Autodesk Inventor part; units mm, degrees
ref_plane "YZ Plane" through (0, 0, 0) normal (1, 0, 0) x (0, 1, 0)
ref_plane "XZ Plane" through (0, 0, 0) normal (0, 1, 0) x (-1, 0, 0)
ref_plane "XY Plane" through (0, 0, 0) normal (0, 0, 1) x (1, 0, 0)
sketch "Sketch1" plane through (0, 0, 0) normal (0, 1, 0) x (-1, 0, 0)
  line L0 (12.7, -31.75) -> (-12.7, -31.75)
  line L1 (-12.7, -31.75) -> (-12.7, 31.75)
  line L2 (-12.7, 31.75) -> (12.7, 31.75)
  line L3 (12.7, 31.75) -> (12.7, -31.75)
  line L4 (12.7, -31.75) -> (-12.7, 31.75) construction
  line L5 (-12.7, -31.75) -> (12.7, 31.75) construction
  line L6 (-5.5118, -31.75) -> (-5.5118, 31.75)
  line L7 (12.7, 0) -> (-12.7, 0)
  circle A0 centre (-5.5118, 24.5618) radius 3.5052
  circle A1 centre (-5.5118, -24.5618) radius 3.5052
  line L8 (88.6284, 0) -> (-89.1716, 0)
  circle A2 centre (-30.9118, 0) radius 3.81
  line L9 (12.7, 31.75) -> (-12.7, 31.75)
  circle A3 centre (-30.9118, 0) radius 10.9982
  point P0 (0, 0)
  dimension "d0" = 25.4
  dimension "d1" = 63.5
  dimension "d2" = 7.1882
  dimension "d3" = 7.1882
  dimension "d4" = 7.0104
  dimension "d5" = 7.62
  dimension "d6" = 177.8
  dimension "d7" = 0
  dimension "d8" = 25.4
  dimension "d10" = 7.1882
extrude "Extrusion1" add sketch "Sketch1" along normal blind 5
sketch "Sketch2" plane through (0, 5, 0) normal (0, 1, 0) x (1, 0, 0)
  line L0 (12.7, -31.75) -> (38.3668, -8.086)
  circle A0 centre (30.9118, 0) radius 10.9982
  circle A1 centre (30.9118, 0) radius 10.9982
  line L1 (-12.7, 31.75) -> (-12.7, -31.75)
  line L2 (-12.7, 0) -> (12.7, 0)
  line L3 (12.7, -31.75) -> (12.7, 31.75)
  line L4 (12.7, 31.75) -> (38.3668, 8.086)
  line L5 (38.3668, 8.086) -> (38.3668, -8.086)
  line L6 (12.7, -31.75) -> (12.7, 31.75)
  point P0 (0, 0)
extrude "Extrusion2" add sketch "Sketch2" against normal up to surface (5 mm away) contours L3 L4 A0 L0 | A0 L5 picked at (33.4709, -2.7618)
sketch "Sketch3" plane through (0, 5, 0) normal (0, 1, 0) x (1, 0, 0)
  line L0 (12.7, 31.75) -> (12.7, -31.75)
  line L1 (12.7, 31.75) -> (-12.7, 31.75)
  line L2 (5.5118, 31.75) -> (5.5118, -31.75)
  line L3 (-12.7, -31.75) -> (12.7, -31.75)
  circle A0 centre (5.5118, 24.5618) radius 4.4958
  line L4 (-12.7, 31.75) -> (-12.7, -31.75)
  line L5 (-12.7, 0) -> (12.7, 0)
  circle A1 centre (5.5118, -24.5618) radius 4.4958
  circle A2 centre (30.9118, 0) radius 3.81
  point P0 (0, 0)
  dimension "d15" = 7.1882
  dimension "d16" = 7.1882
  dimension "d17" = 8.9916
  dimension "d18" = 25.4
  dimension "d19" = 7.62
extrude "Extrusion3" cut sketch "Sketch3" against normal through all contours A0 L2 | L2 A0 | A1 L2 | L2 A1 | A2
properties part number "Foundation 6_2"
Could you check a few things on this model? Use its own coordinates, in mm. Coordinates: 2 decimals unless noted, no trailing zeros. Order: outer loops, then holes, each group sorted by start corner. A loop starts at its lowest first (then second) coordinate and runs counter-clockwise, first axis right, second up. Notation, with made-up numbers: M 21.25,2 L 74.25,2 A22 cw 74.25,14 Z; hole C 69,79 d7. An arc over 180 degrees is marked long. Use one line per item in the form item = value. Start each with the question number.
1. Suppose I cut it at C-C on y = 1.2. Write out the boundary of the cut face in (x, z), then the cut area to 3 significant figures.
2. Suppose I cut it at D-D on x = 14.5. Write out the boundary of the cut face in (y, z).
3. For pin 1 (2 mm diameter, centred on x = 24, y = 1, fed in from -Z); pin 2 (4.5 mm diameter, centred on x = 30.91, z = 0, fed in from +Y), each with a flat end and sliding along its axis, tell me the tip position at first contact or that it passes through.
4. Please list where these lines run through material, in increasing order: line 1 (Z direction, x = 8.5, y = 0.4); line 2 (X direction, y = 4.3, z = -3); line 3 (X direction, y = 3.2, z = -26.5).
5. Suppose I cut it at A-A on x = 3. Write out the boundary of the cut face in (y, z).
6. Suppose I cut it at B-B on z = 0. Write out the boundary of the cut face in (x, y).
7. We'd pull the mould along X, two halves only. Please class faces 1 (the flat face through (-12.7, 2, 0)), 2 (the flat face through (25.354, 2.535, 20.084)), 3 (the cylindrical face through (27.105, 2.535, -0.168)): +X half, -X half, draft (parallel to the pull), parting line (faces both ways), or undercut.
Geometry says:
q1.outline = M -12.7,-31.75 L 12.7,-31.75 L 38.37,-8.09 A11 ccw 38.37,8.09 L 12.7,31.75 L -12.7,31.75 Z; hole C 5.51,-24.56 d8.99; hole C 5.51,24.56 d8.99; hole C 30.91,0 d7.62
q1.area = 2,500 mm^2
q2.outline = M 0,-30.09 L 5,-30.09 L 5,30.09 L 0,30.09 Z
q3.pin_1 = -22.25
q3.pin_2 = through
q4.line_1 = -31.75 to -27.92, -21.2 to 21.2, 27.92 to 31.75
q4.line_2 = -12.7 to 28.56, 33.26 to 41.49
q4.line_3 = -12.7 to 1.46, 9.57 to 18.39
q5.outline = M 0,-31.75 L 5,-31.75 L 5,-28.29 L 0,-28.29 Z; M 0,-20.83 L 5,-20.83 L 5,20.83 L 0,20.83 Z; M 0,28.29 L 5,28.29 L 5,31.75 L 0,31.75 Z
q6.outline = M -12.7,0 L 27.1,0 L 27.1,5 L -12.7,5 Z; M 34.72,0 L 41.91,0 L 41.91,5 L 34.72,5 Z
q7.face_1 = -X half
q7.face_2 = +X half
q7.face_3 = undercut
